from build123d import *

# Parameters (mm, degrees)
SKETCH1_R                      = 7.266716582
BASE_FLANGE1_DEPTH             = 1.5
EDGE_FLANGE1_STRIP_W           = 7.4732
EDGE_FLANGE1_STRIP_H           = 1.5
EDGE_FLANGE1_STRIP_CUT_DEPTH   = 12
EDGE_FLANGE1_STRIP_2_W         = 7.4732
EDGE_FLANGE1_STRIP_2_H         = 1.5
EDGE_FLANGE1_STRIP_CUT_2_DEPTH = 12
EDGE_FLANGE1_DEPTH             = 12
EDGE_FLANGE1_BEND_DEPTH        = 12
SKETCH9_R                      = 1.5
CUT_EXTRUDE1_DEPTH             = 35.286317994
FILLET1_R                      = 2
EDGE_FLANGE3_STRIP_W           = 7.4732
EDGE_FLANGE3_STRIP_H           = 1.5
EDGE_FLANGE3_STRIP_CUT_DEPTH   = 9.2634
EDGE_FLANGE3_DEPTH             = 9.2634
FILLET2_R                      = 2.54
FILLET2_OF_MIRROR1_R           = 2.54
SKETCH20_R                     = 1.5875
CUT_EXTRUDE3_DEPTH             = 2.54


# Sheet-metal steps are written as plain solids
with BuildPart() as part:
    # Sketch1 → Base-Flange1 (new body)
    with BuildSketch(Plane.XY):
        Polygon((-9, -16.31875), (9, -16.31875), (9, -4.31875), (12.5, -4.31875), (12.5, 10), (-12.5, 10), (-12.5, -4.31875), (-9, -4.31875), align=None)
        Circle(SKETCH1_R, mode=Mode.SUBTRACT)
    extrude(amount=BASE_FLANGE1_DEPTH)

    # Edge-Flange1 strip (across the edge) → Edge-Flange1 strip cut (cut)
    with BuildSketch(Plane(origin=(-9, -4.31875, 1.5), x_dir=(1, 0, 0), z_dir=(0, -1, 0))):
        with Locations((-3, -0.75)):
            Rectangle(EDGE_FLANGE1_STRIP_W, EDGE_FLANGE1_STRIP_H)
    extrude(amount=EDGE_FLANGE1_STRIP_CUT_DEPTH, mode=Mode.SUBTRACT)

    # Edge-Flange1 strip 2 (across the edge) → Edge-Flange1 strip cut 2 (cut)
    with BuildSketch(Plane(origin=(9, -16.31875, 1.5), x_dir=(-1, 0, 0), z_dir=(0, 1, 0))):
        with Locations((-3, -0.75)):
            Rectangle(EDGE_FLANGE1_STRIP_2_W, EDGE_FLANGE1_STRIP_2_H)
    extrude(amount=EDGE_FLANGE1_STRIP_CUT_2_DEPTH, mode=Mode.SUBTRACT)

    # Edge-Flange1 section (across the edge) → Edge-Flange1 (add)
    with BuildSketch(Plane(origin=(-9, -4.31875, 1.5), x_dir=(1, 0, 0), z_dir=(0, -1, 0))):
        with BuildLine():
            Line((-1.5, 0.7366), (-1.5, 18))
            Line((-1.5, 18), (0, 18))
            Line((0, 18), (0, 0.7366))
            ThreePointArc((0, 0.7366), (0.215745145, 0.215745145), (0.7366, 0))
            Line((0.7366, 0), (0.7366, -1.5))
            ThreePointArc((0.7366, -1.5), (-0.844915027, -0.844915027), (-1.5, 0.7366))
        make_face()
    extrude(amount=EDGE_FLANGE1_DEPTH)

    # Edge-Flange1 section 2 (across the edge) → Edge-Flange1 bend (add)
    with BuildSketch(Plane(origin=(9, -16.31875, 1.5), x_dir=(-1, 0, 0), z_dir=(0, 1, 0))):
        with BuildLine():
            Line((-1.5, 0.7366), (-1.5, 18))
            Line((-1.5, 18), (0, 18))
            Line((0, 18), (0, 0.7366))
            ThreePointArc((0, 0.7366), (0.215745145, 0.215745145), (0.7366, 0))
            Line((0.7366, 0), (0.7366, -1.5))
            ThreePointArc((0.7366, -1.5), (-0.844915027, -0.844915027), (-1.5, 0.7366))
        make_face()
    extrude(amount=EDGE_FLANGE1_BEND_DEPTH)

    # Sketch9 → Cut-Extrude1 (cut, through all)
    with BuildSketch(Plane(origin=(10.5, 0, 0), x_dir=(0, 0, -1), z_dir=(1, 0, 0))):
        with Locations((-15.2366, -10.31875)):
            Circle(SKETCH9_R)
    extrude(amount=-CUT_EXTRUDE1_DEPTH, mode=Mode.SUBTRACT)

    # Fillet1
    fillet1_edges = [part.edges().sort_by_distance(p)[0] for p in [
        (-12.5, -4.31875, 0.75),
        (-12.5, 10, 0.75),
        (12.5, 10, 0.75),
        (12.5, -4.31875, 0.75),
        (-9.75, -4.31875, 19.5),
        (-9.75, -16.31875, 19.5),
        (9.75, -16.31875, 19.5),
        (9.75, -4.31875, 19.5),
    ]]
    fillet(fillet1_edges, radius=FILLET1_R)

    # Edge-Flange3 strip (across the edge) → Edge-Flange3 strip cut (cut)
    with BuildSketch(Plane(origin=(10.5, -4.31875, 5.2366), x_dir=(0, -1, 0), z_dir=(0, 0, 1))):
        with Locations((-1.5, -0.75)):
            Rectangle(EDGE_FLANGE3_STRIP_W, EDGE_FLANGE3_STRIP_H)
    edge_flange3_strip_cut = extrude(amount=EDGE_FLANGE3_STRIP_CUT_DEPTH, mode=Mode.SUBTRACT)

    # Edge-Flange3 section (across the edge) → Edge-Flange3 (add)
    with BuildSketch(Plane(origin=(10.5, -4.31875, 5.2366), x_dir=(0, -1, 0), z_dir=(0, 0, 1))):
        with BuildLine():
            Line((0, 0.7366), (0, 6.2766))
            Line((0, 6.2766), (1.5, 6.2766))
            Line((1.5, 6.2766), (1.5, 0.7366))
            ThreePointArc((1.5, 0.7366), (1.715745145, 0.215745145), (2.2366, 0))
            Line((2.2366, 0), (2.2366, -1.5))
            ThreePointArc((2.2366, -1.5), (0.655084973, -0.844915027), (0, 0.7366))
        make_face()
    edge_flange3 = extrude(amount=EDGE_FLANGE3_DEPTH)

    # Fillet2
    fillet2_edges = [part.edges().sort_by_distance(p)[0] for p in [
        (16.7766, -5.06875, 5.2366),
        (16.7766, -5.06875, 14.5),
    ]]
    fillet(fillet2_edges, radius=FILLET2_R)

    # Mirror1: Edge-Flange3 strip cut, Edge-Flange3 across plane
    add(edge_flange3_strip_cut.mirror(Plane(origin=(0, 0, 0), x_dir=(0, 0, 1), z_dir=(1, 0, 0))), mode=Mode.SUBTRACT)
    add(edge_flange3.mirror(Plane(origin=(0, 0, 0), x_dir=(0, 0, 1), z_dir=(1, 0, 0))))

    # Fillet2 of Mirror1
    fillet2_of_mirror1_edges = [part.edges().sort_by_distance(p)[0] for p in [
        (-16.7766, -5.06875, 5.2366),
        (-16.7766, -5.06875, 14.5),
    ]]
    fillet(fillet2_of_mirror1_edges, radius=FILLET2_OF_MIRROR1_R)

    # Sketch20 → Cut-Extrude3 (cut)
    with BuildSketch(Plane(origin=(0, -4.31875, 0), x_dir=(1, 0, 0), z_dir=(0, 1, 0))):
        with Locations(Location((14.0066, -9.8683, 0), (0, 0, 180))):
            Circle(SKETCH20_R)
        with Locations(Location((-14.0066, -9.8683, 0), (0, 0, 180))):
            Circle(SKETCH20_R)
    extrude(amount=-CUT_EXTRUDE3_DEPTH, mode=Mode.SUBTRACT)


solid = part.part
Source: CAD feature listing. Evaluate the final solid. Frame: model axes, mm. A direction names the side the tool comes from. Coordinates: 2 decimals unless noted, no trailing zeros. Loops run counter-clockwise (first coordinate to the right, second up) from the corner with the lowest first, then second, coordinate; pieces in that order, holes last. Notation, with made-up numbers: (49, -30.5) -> (107, -30.5) arc R21 ccw to (107, -23.5) -> close; hole circle Ø9 at (-16, -40). An arc over 180 degrees is marked (long way). Answer in a Markdown table with one row per item. Add a question column.
Q1. Ray query, line 1 along X through (y, z) = (-13, 3.5); line 2 along Z through (x, y) = (5.5, -12); line 3 along Y through (x, z) = (9.5, 2.5). Return the intervals inside material, ascending.
Q2. Reachability of faces 1 (the face through (10, -4.319, 0.5)), 2 (the face through (-12, -5.819, 10)), 3 (the face through (-9.83, -10.23, 0.64)), 4 (the face through (-12, -5, 14.5)), 5 (the face through (9.64, -4.99, 9.8)) from +Z, -Z, +X, -X, +Y, -Y: full face, straight path, thin tool, end or side. Return the list, or none.
Q3. Section B-B on y = 0. Return the cut outline in (x, z), and give its area (3 significant figures).
Q4. Section A-A on x = 0. Return the cut outline in (y, z), and give its area (3 significant figures).
Q5. Contact query for flat-ended pins moving along their axis: pin 1 Ø2.5 at (y, z) = (-10.32, 15.24) entering from +X; pin 2 Ø10 at (y, z) = (-11, 8) entering from +X; pin 3 Ø9.5 at (y, z) = (-12, 7.5) entering from +X; pin 4 Ø0.8 at (x, z) = (9.5, 16.5) entering from +Y. Output: stop coordinate, or through.
Q6. Pull-direction query (Y, two-part tool) for faces 6 (the face through (11.93, 9.4, 0.76)), 7 (the face through (-10, -4.319, 0.4)), 8 (the face through (-10.5, -10, 11)), 9 (the face through (-9.74, -8.83, 15.43)); classes: pulls with the +Y half, pulls with the -Y half, needs draft (parallel to the pull), parting line crosses it, or undercut.
Q7. Section C-C on y = -13.75. Return the cut outline in (x, z).
Computed values:
| question | item | result |
|---|---|---|
| 1 | line 1 | x = -10.5 to -9, 9 to 10.5 |
| 1 | line 2 | z = 0 to 1.5 |
| 1 | line 3 | y = -16.32 to -4.32 |
| 2 | face 1 | -Z, +X, -Y |
| 2 | face 2 | +Z, -Z, -X, -Y |
| 2 | face 3 | -Z, -X, -Y |
| 2 | face 4 | +Z, -X, +Y, -Y |
| 2 | face 5 | +Y |
| 3 | outline | (-12.5, 0) -> (-7.27, 0) -> (-7.27, 1.5) -> (-12.5, 1.5) -> close; (7.27, 0) -> (12.5, 0) -> (12.5, 1.5) -> (7.27, 1.5) -> close |
| 3 | area | 15.7 mm^2 |
| 4 | outline | (-16.32, 0) -> (-7.27, 0) -> (-7.27, 1.5) -> (-16.32, 1.5) -> close; (7.27, 0) -> (10, 0) -> (10, 1.5) -> (7.27, 1.5) -> close |
| 4 | area | 17.7 mm^2 |
| 5 | pin 1 | passes through |
| 5 | pin 2 | stops at x = 10.75 |
| 5 | pin 3 | stops at x = 10.5 |
| 5 | pin 4 | stops at y = -4.32 |
| 6 | face 6 | pulls with the +Y half |
| 6 | face 7 | pulls with the -Y half |
| 6 | face 8 | needs draft |
| 6 | face 9 | undercut |
| 7 | outline | (-10.5, 2.24) arc R2.24 ccw to (-8.26, 0) -> (8.26, 0) arc R2.24 ccw to (10.5, 2.24) -> (10.5, 19.5) -> (9, 19.5) -> (9, 2.24) arc R0.74 cw to (8.26, 1.5) -> (-8.26, 1.5) arc R0.74 cw to (-9, 2.24) -> (-9, 19.5) -> (-10.5, 19.5) -> close |
